from build123d import *

# Parameters (mm, degrees)
ESBO_O1_R                = 6.3
RESSALTO_EXTRUS_O1_DEPTH = 0.5
ESBO_O10_R               = 5.5
RESSALTO_EXTRUS_O4_DEPTH = 1
ESBO_O11_R               = 6.3
RESSALTO_EXTRUS_O5_DEPTH = 0.5
CORTE_EXTRUS_O1_REACH    = 4
ESBO_O12_R               = 0.675


with BuildPart() as part:
    # Esboço1 → Ressalto-extrusão1 (new body)
    with BuildSketch(Plane(origin=(0, 0, 0), x_dir=(1, 0, 0), z_dir=(0, 1, 0))):
        Circle(ESBO_O1_R)
    extrude(amount=RESSALTO_EXTRUS_O1_DEPTH)

    # Esboço10 → Ressalto-extrusão4 (add)
    with BuildSketch(Plane(origin=(0, 0.5, 0), x_dir=(1, 0, 0), z_dir=(0, 1, 0))):
        Circle(ESBO_O10_R)
    extrude(amount=RESSALTO_EXTRUS_O4_DEPTH)

    # Esboço11 → Ressalto-extrusão5 (add)
    with BuildSketch(Plane(origin=(0, 1.5, 0), x_dir=(1, 0, 0), z_dir=(0, 1, 0))):
        Circle(ESBO_O11_R)
    extrude(amount=RESSALTO_EXTRUS_O5_DEPTH)

    # Esboço12 → Corte-extrusão1 (cut, up to next)
    with BuildSketch(Plane.XZ, mode=Mode.PRIVATE) as corte_extrus_o1_sk1:
        Circle(ESBO_O12_R)
    corte_extrus_o1_tool1 = extrude(corte_extrus_o1_sk1.sketch, amount=-CORTE_EXTRUS_O1_REACH, mode=Mode.PRIVATE) & part.part
    add(corte_extrus_o1_tool1.solids().sort_by_distance((0, 0, 0))[0], mode=Mode.SUBTRACT)


solid = part.part
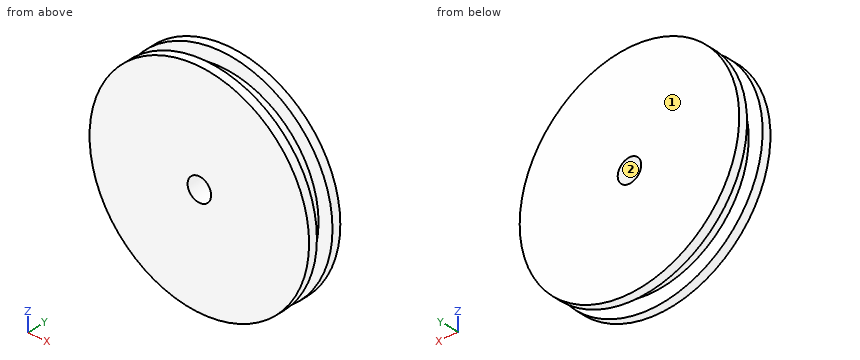
Geometry: final body of the model. Coordinates: model frame, mm. Face numbers are marked on the shaded views. Give positions to 0.01 mm unless a question says otherwise; leave off trailing zeros. Write each loop counter-clockwise with the first axis right and the second up, starting at its lowest first coordinate (ties: lowest second). Pieces come first, ordered by that corner, then holes. Notation, with made-up numbers: (64, -25.75) - (87, -25.75) arc R25 cw to (87, 4.25) - close; hole circle Ø3 at (51.5, 44). An arc over 180 degrees is marked (long way). Return JSON: item names as keys, results as strings. Group by question number.
1) Section B-B on x = 0. Return the cut outline in (y, z) (3 decimals), plus the area to 3 significant figures.
2) First-contact query: P1, Ø1, axis at x = 4, y = 0.5, coming from the +Z side. Flat tip, straight axial feed; report the tip coordinate or a pass-through.
3) Line query: line 1 (Z direction, x = 0, y = 0.6) (3 decimals); line 2 (Y direction, x = 5.75, z = 0.25); line 3 (Z direction, x = 0, y = 1.6) (3 decimals). Output: solid intervals per line, ascending.
4) Section C-C on y = 1. Return the cut outline in (x, z) (3 decimals).
5) Section D-D on x = 4.75. Return the cut outline in (y, z), plus the area to 3 significant figures.
6) Mould query, pull axis Z, two halves, no side actions, for the marked faces 1 and 2. Classes: released by +Z, released by -Z, zero draft, split by the parting line, or undercut.
7) Section A-A on z = 0. Return the cut outline in (x, y) (3 decimals), plus the area to 3 significant figures.
Filled in:
{
 "1": {"outline": "(0, -6.3) - (0.5, -6.3) - (0.5, -5.5) - (1.5, -5.5) - (1.5, -6.3) - (2, -6.3) - (2, -0.675) - (0, -0.675) - close; (0, 0.675) - (2, 0.675) - (2, 6.3) - (1.5, 6.3) - (1.5, 5.5) - (0.5, 5.5) - (0.5, 6.3) - (0, 6.3) - close", "area": "20.9 mm^2"},
 "2": {"P1": "stops at z = 5.24"},
 "3": {"line 1": "z = -5.5 to -0.675, 0.675 to 5.5", "line 2": "y = 0 to 0.5, 1.5 to 2", "line 3": "z = -6.3 to -0.675, 0.675 to 6.3"},
 "4": {"outline": "circle Ø11 at (0, 0); hole circle Ø1.35 at (0, 0)"},
 "5": {"outline": "(0, -4.14) - (0.5, -4.14) - (0.5, -2.77) - (1.5, -2.77) - (1.5, -4.14) - (2, -4.14) - (2, 4.14) - (1.5, 4.14) - (1.5, 2.77) - (0.5, 2.77) - (0.5, 4.14) - (0, 4.14) - close", "area": "13.8 mm^2"},
 "6": {"face 1": "zero draft", "face 2": "undercut"},
 "7": {"outline": "(-6.3, 0) - (-0.675, 0) - (-0.675, 2) - (-6.3, 2) - (-6.3, 1.5) - (-5.5, 1.5) - (-5.5, 0.5) - (-6.3, 0.5) - close; (0.675, 0) - (6.3, 0) - (6.3, 0.5) - (5.5, 0.5) - (5.5, 1.5) - (6.3, 1.5) - (6.3, 2) - (0.675, 2) - close", "area": "20.9 mm^2"}
}
